Check sheet for the drawn part. Datum: minimum x, y, z corner. Units: mm. A direction names the side the tool comes from. Give positions to 0.01 mm unless a question says otherwise; leave off trailing zeros. Loops run counter-clockwise (first coordinate to the right, second up) from the corner with the lowest first, then second, coordinate; pieces in that order, holes last. Notation, with made-up numbers: (38.25, -4) - (92.25, -4) arc R25 cw to (92.25, 22) - close; hole circle Ø8 at (88.5, -28). An arc over 180 degrees is marked (long way). Use one line per item in the form item = value.
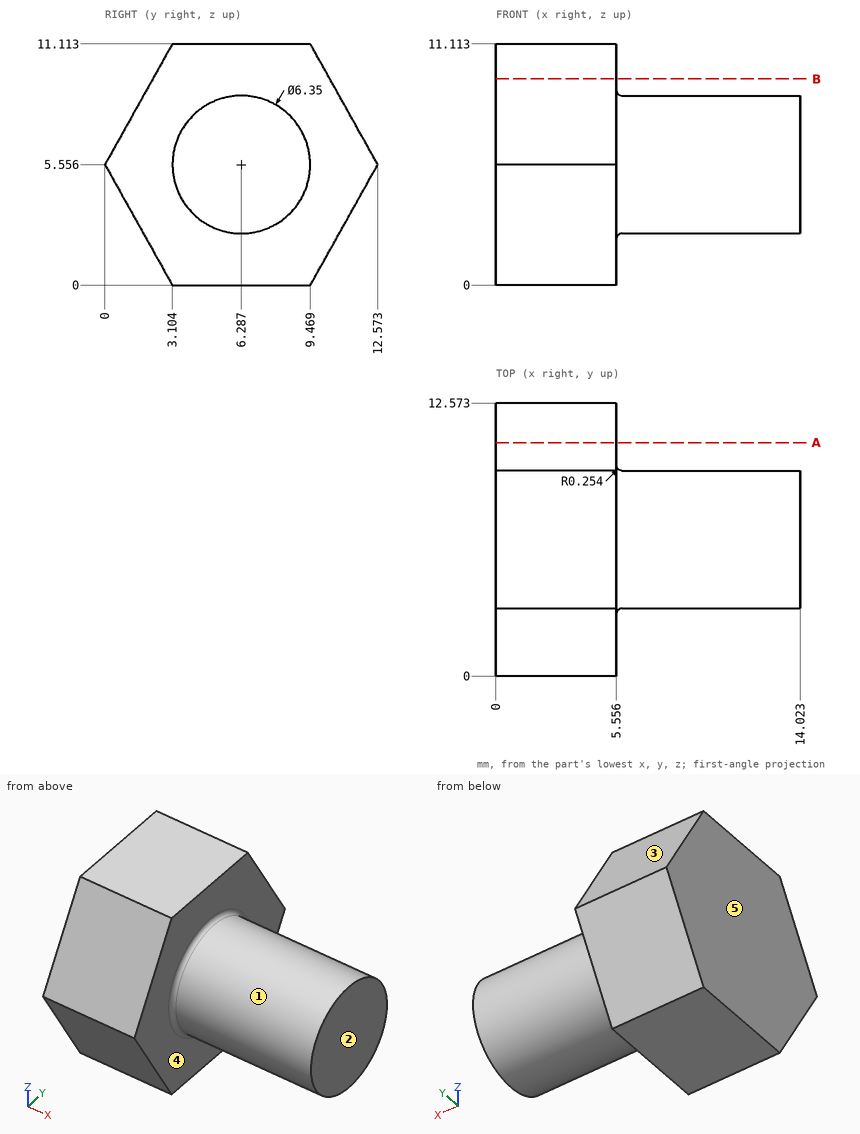
Item 1: Mould release check, pull along Y, two halves, no side actions. Record for the marked faces 1, 2 and 3: released by +Y, released by -Y, zero draft, split by the parting line, or undercut.
Answer block:
face_1 = split by the parting line
face_2 = zero draft
face_3 = released by +Y
Item 2: Access from +Z, -Z, +X, -X, +Y, -Y to the whole of each face (thin tool, end or side, straight path). Record for the marked faces 4 and 5.
Answer block:
face_4 = +X
face_5 = +Z, -Z, -X, +Y, -Y
Item 3: Section check B-B on z = 9.5. Record the boundary of the cut face in (x, y).
Answer block:
outline = (0, 2.2) - (5.56, 2.2) - (5.56, 10.37) - (0, 10.37) - close
Item 4: Gauge pin test, flat ends, axial feed: P1, Ø1.5, axis at x = 7, z = 6, coming from the -Y side; P2, Ø1.5, axis at x = 10.5, z = 2.5, coming from the +Y side; P3, Ø4, axis at x = 5.5, z = 8, coming from the +Y side (1 decimal). Record the tip position at first contact, or that the pin passes through.
Answer block:
P1 = 3.11
P2 = 8.47
P3 = 12.3
Item 5: Thickness scan on L1, parallel to X at y = 12, z = 5.25; L2, parallel to Z at x = 4, y = 2.25 (1 decimal); L3, parallel to Y at x = 6.5, z = 7.5 (1 decimal). Record the ranges inside material, lowest first.
Answer block:
L1 = 0 to 5.56
L2 = 1.5 to 9.6
L3 = 3.8 to 8.8
Item 6: Section check A-A on y = 10.75. Record the boundary of the cut face in (x, z).
Answer block:
outline = (0, 2.29) - (5.56, 2.29) - (5.56, 8.82) - (0, 8.82) - close
